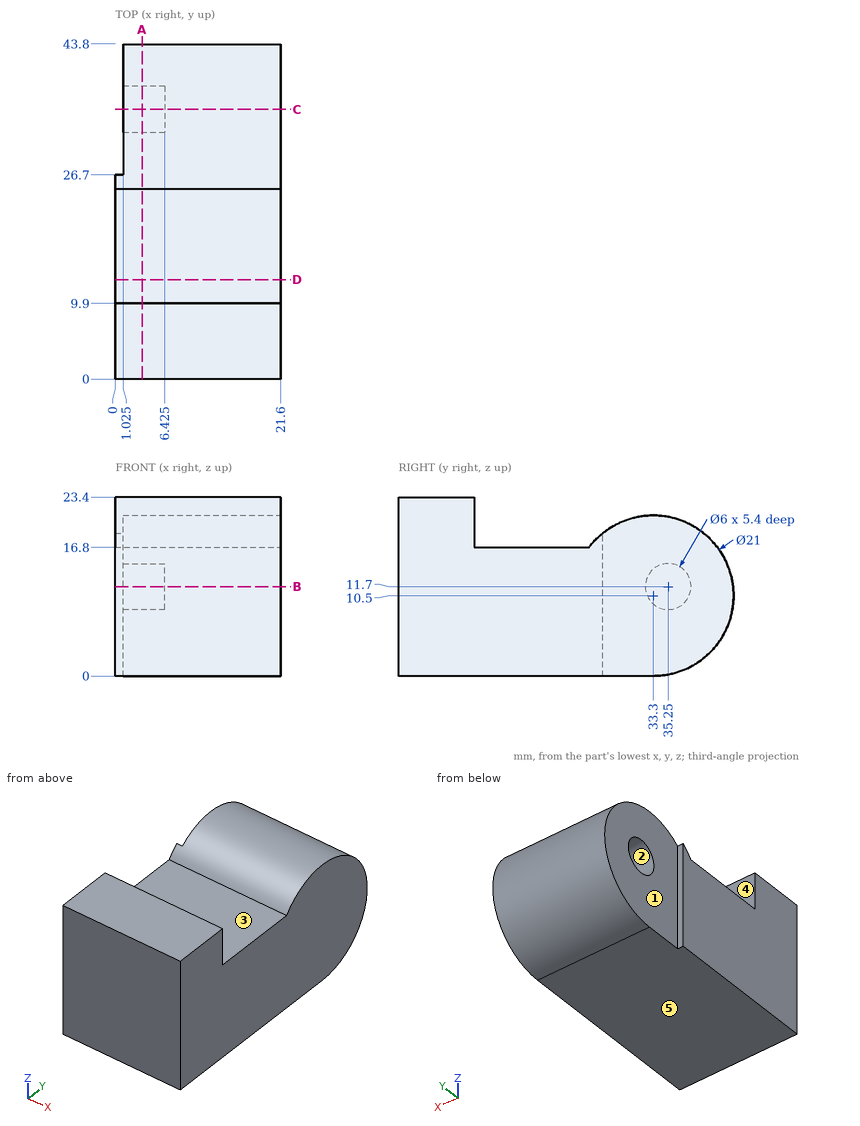
Job drawing, mm, ordinate dimensions from the low corner. One solid piece. A direction names the side the tool comes from. Give positions to 0.01 mm unless a question says otherwise; leave off trailing zeros. Write each loop counter-clockwise with the first axis right and the second up, starting at its lowest first coordinate (ties: lowest second). Pieces come first, ordered by that corner, then holes. Notation, with made-up numbers: M 67,12.25 L 108,12.25 A19 cw 108,49.25 Z; hole C 72.5,84 d11. An arc over 180 degrees is marked long. Put each result on its own line as item: value. Start each with the question number.
(1) Probe L1, parallel to X at y = 40.5, z = 3.5 (3 decimals); L2, parallel to Y at x = 4.35, z = 11.7; L3, parallel to Y at x = 7.5, z = 17.75. List the from-to ranges inside material, lowest first.
(2) Band-saw the part on A-A, the plane x = 3.5. Write the cut outline in (y, z), and give its area (3 significant figures).
(3) Band-saw the part on C-C, the plane y = 35.25. Write the cut outline in (x, z) (3 decimals), and give its area (3 significant figures).
(4) Band-saw the part on D-D, the plane y = 13. Write the cut outline in (x, z), and give its area (3 significant figures).
(5) Flat gauge pins, fed straight in: pin 1 Ø4.5 at (x, y) = (6.5, 14) entering from +Z; pin 2 Ø5 at (y, z) = (37, 7.5) entering from -X (3 decimals); pin 3 Ø5 at (x, y) = (10, 37) entering from +Z. Where does each tip first touch, or does it go through?
(6) Mould opens along Z. For the marked faces 1, 2 and 3 say: +Z half, -Z half, draft (parallel to the pull), parting line (faces both ways), or undercut.
(7) Band-saw the part on B-B, the plane z = 11.7. Write the cut outline in (x, y) (3 decimals), and give its area (3 significant figures).
(8) Which spindle directions (+Z, -Z, +X, -X, +Y, -Y) get a long thin tool onto all of the face, cutting with end or side? Do the marked faces 4 and 5. Say none if no direction does.
Response values:
1. L1: x = 1.025 to 21.6
1. L2: y = 0 to 32.25, 38.25 to 43.73
1. L3: y = 0 to 9.9, 25.7 to 40.9
2. outline: M 0,0 L 33.3,0 A10.5 ccw long 24.9,16.8 L 9.9,16.8 L 9.9,23.4 L 0,23.4 Z; hole C 35.25,11.7 d6
2. area: 794 mm2
3. outline: M 1.025,0.183 L 21.6,0.183 L 21.6,20.817 L 1.025,20.817 L 1.025,14.7 L 6.425,14.7 L 6.425,8.7 L 1.025,8.7 Z
3. area: 392 mm2
4. outline: M 0,0 L 21.6,0 L 21.6,16.8 L 0,16.8 Z
4. area: 363 mm2
5. pin 1: stops at z = 16.8
5. pin 2: stops at x = 1.025
5. pin 3: stops at z = 20.93
6. face 1: draft
6. face 2: undercut
6. face 3: +Z half
7. outline: M 0,0 L 21.6,0 L 21.6,43.731 L 1.025,43.731 L 1.025,38.25 L 6.425,38.25 L 6.425,32.25 L 1.025,32.25 L 1.025,26.7 L 0,26.7 Z
7. area: 895 mm2
8. face 4: +Z, +X, -X
8. face 5: -Z, +X, -X, +Y, -Y
